Autodesk Inventor part; units mm, degrees
ref_plane "YZ Plane" through (0, 0, 0) normal (1, 0, 0) x (0, 1, 0)
ref_plane "XZ Plane" through (0, 0, 0) normal (0, 1, 0) x (-1, 0, 0)
ref_plane "XY Plane" through (0, 0, 0) normal (0, 0, 1) x (1, 0, 0)
sketch "Sketch1" plane through (0, 0, 0) normal (0, 1, 0) x (-1, 0, 0)
  line L0 (200.4562, 91.842) -> (79.4562, 91.842)
  line L1 (79.4562, 91.842) -> (79.4562, 63.142)
  line L2 (79.4562, 63.142) -> (200.4562, 63.142)
  line L3 (200.4562, 63.142) -> (200.4562, 91.842)
  point P0 (0, 0)
  dimension "d0" = 121
  dimension "d1" = 28.7
extrude "Extrusion1" add sketch "Sketch1" along normal blind 26.8
sketch "Sketch2" plane through (-79.4562, 0, 91.842) normal (1, 0, 0) x (0, 0, -1)
  line L0 (4.95, 3) -> (23.75, 3)
  line L1 (24.75, 4) -> (24.75, 22.8)
  line L2 (23.75, 23.8) -> (4.95, 23.8)
  line L3 (3.95, 22.8) -> (3.95, 4)
  line L4 (28.7, 0) -> (28.7, 26.8)
  line L5 (0, 0) -> (0, 26.8)
  line L6 (0, 26.8) -> (28.7, 26.8)
  arc A0 (24.75, 22.8) -> (23.75, 23.8) centre (23.75, 22.8) ccw
  arc A1 (23.75, 3) -> (24.75, 4) centre (23.75, 4) ccw
  arc A2 (3.95, 4) -> (4.95, 3) centre (4.95, 4) ccw
  arc A3 (4.95, 23.8) -> (3.95, 22.8) centre (4.95, 22.8) ccw
  line L7 (0, 0) -> (28.7, 0)
  point P0 (91.842, 0)
  point P1 (3.95, 3)
  point P2 (24.75, 23.8)
  point P3 (3.95, 23.8)
  dimension "d4" = 20.8
  dimension "d5" = 20.8
  dimension "d7" = 3.95
  dimension "d8" = 3
  dimension "d9" = 1
  dimension "d137" = 3.95
  dimension "d138" = 3
extrude "Extrusion2" cut sketch "Sketch2" against normal blind 121 contours A2 L3 A3 L2 A0 L1 A1 L0
sketch "Sketch3" plane through (0, 0, 0) normal (0, -1, 0) x (1, 0, 0)
  line L0 (-200.4562, 63.142) -> (-200.4562, 91.842)
  line L1 (-200.4562, 91.842) -> (-79.4562, 91.842)
  line L2 (-79.4562, 63.142) -> (-200.4562, 63.142)
  circle A0 centre (-188.2062, 77.492) radius 9.25
  line L3 (-79.4562, 91.842) -> (-79.4562, 63.142)
  point P0 (0, 0)
  dimension "d20" = 14.35
  dimension "d21" = 18.5
  dimension "d287" = 12.25
hole "Hole1" at (-188.2062, 0, 77.492) direction (0, 1, 0) diameter 18.5 depth 5
sketch "Sketch4" plane through (0, 26.8, 0) normal (0, 1, 0) x (1, 0, 0)
  line L0 (-85.9562, -84.142) -> (-193.9562, -84.142)
  line L1 (-193.9562, -84.142) -> (-193.9562, -70.642)
  line L2 (-193.9562, -70.642) -> (-85.9562, -70.642)
  line L3 (-85.9562, -70.642) -> (-85.9562, -84.142)
  line L4 (-79.4562, -91.842) -> (-79.4562, -63.142)
  line L5 (-200.4562, -63.142) -> (-200.4562, -91.842)
  point P0 (0, 0)
  point P1 (-79.4562, -86.142)
  point P2 (-79.4562, -65.142)
  point P3 (-179.4562, -65.142)
  point P4 (-179.4562, -86.142)
  point P5 (-200.4562, -91.842)
  point P6 (-79.4562, -87.892)
  dimension "d30" = 6.5
  dimension "d31" = 6.5
  dimension "d32" = 13.5
  dimension "d41" = 3.75
extrude "Extrusion3" cut sketch "Sketch4" against normal blind 5
sketch "Sketch5" plane through (0, 26.8, 0) normal (0, 1, 0) x (1, 0, 0)
  line L0 (-79.4562, -91.842) -> (-79.4562, -63.142)
  line L1 (-200.4562, -63.142) -> (-200.4562, -91.842)
  line L2 (-79.4562, -91.842) -> (-200.4562, -91.842)
  line L3 (-200.4562, -91.842) -> (-200.4562, -88.442)
  line L4 (-200.4562, -88.442) -> (-79.4562, -88.442)
  line L5 (-79.4562, -88.442) -> (-79.4562, -91.842)
  line L6 (-79.4562, -63.142) -> (-200.4562, -63.142)
  line L7 (-200.4562, -63.142) -> (-200.4562, -66.142)
  line L8 (-200.4562, -66.142) -> (-79.4562, -66.142)
  line L9 (-79.4562, -66.142) -> (-79.4562, -63.142)
  line L10 (-79.4562, -63.142) -> (-200.4562, -63.142)
  line L11 (-79.4562, -87.892) -> (-79.4562, -87.642)
  line L12 (-79.4562, -87.642) -> (-79.4562, -81.492)
  point P0 (0, 0)
  point P1 (-79.4562, -66.142)
  dimension "d38" = 3.4
  dimension "d39" = 3
  dimension "d40" = 0
  dimension "d42" = 22.3
  dimension "d288" = 0.25
  dimension "d289" = 6.15
extrude "Extrusion4" add sketch "Sketch5" along normal blind 8 contours L2 L1 L4 L0 | L1 L6 L0 L8
sketch "Sketch6" plane through (0, 34.8, 0) normal (0, 1, 0) x (1, 0, 0)
  line L0 (-200.4562, -91.842) -> (-79.4562, -91.842)
  line L1 (-200.4562, -66.142) -> (-200.4562, -88.442)
  line L2 (-79.4562, -91.842) -> (-200.4562, -91.842)
  line L3 (-200.4562, -91.842) -> (-200.4562, -84.142)
  line L4 (-200.4562, -84.142) -> (-79.4562, -84.142)
  line L5 (-79.4562, -84.142) -> (-79.4562, -91.842)
  line L6 (-79.4562, -63.142) -> (-200.4562, -63.142)
  line L7 (-79.4562, -63.142) -> (-200.4562, -63.142)
  line L8 (-200.4562, -63.142) -> (-200.4562, -70.642)
  line L9 (-200.4562, -70.642) -> (-79.4562, -70.642)
  line L10 (-79.4562, -70.642) -> (-79.4562, -63.142)
  line L11 (-85.9562, -84.142) -> (-193.9562, -84.142)
  line L12 (-193.9562, -70.642) -> (-85.9562, -70.642)
  point P0 (0, 0)
  point P1 (-200.4562, -91.842)
  dimension "d45" = 0
  dimension "d46" = 0
extrude "Extrusion5" add sketch "Sketch6" along normal blind 3
sketch "Sketch11" plane through (-79.4562, 0, 63.142) normal (0, 0, -1) x (-1, 0, 0)
  line L0 (172.6, 9.3) -> (0, 9.3)
  line L1 (0, 9.3) -> (0, 28.3)
  line L2 (0, 28.3) -> (172.6, 28.3)
  line L3 (172.6, 28.3) -> (172.6, 9.3)
  line L4 (0, 37.8) -> (121, 37.8)
  line L5 (0, 0) -> (0, 37.8)
  line L6 (0, 0) -> (121, 0)
  line L7 (0, 28.3) -> (0, 49.8)
  line L8 (0, 34.8) -> (121, 34.8)
  line L9 (121, 0) -> (121, 37.8)
  point P0 (-79.4562, 0)
  point P1 (0, 3)
  dimension "d97" = 0
  dimension "d105" = 12
  dimension "d110" = 9.5
  dimension "d111" = 21.5
  dimension "d113" = 19
  dimension "d114" = 9.3
  dimension "d174" = 51.6
extrude "Extrusion9" add sketch "Sketch11" along normal blind 26.5 contours L0 L9 L2 L3 | L0 L1 L2 L9
sketch "Sketch12" plane through (-252.0562, 28.3, 63.142) normal (0, 1, 0) x (1, 0, 0)
  line L0 (51.6, 3.25) -> (10.1, 3.25)
  line L1 (10.1, 3.25) -> (10.1, 23.25)
  line L2 (10.1, 23.25) -> (51.6, 23.25)
  line L3 (51.6, 23.25) -> (51.6, 3.25)
  line L4 (0, 0) -> (51.6, 0)
  line L5 (0, 26.5) -> (172.6, 26.5)
  line L6 (0, 0) -> (0, 26.5)
  line L7 (51.6, 0) -> (51.6, -7.5)
  line L8 (172.6, 0) -> (51.6, 0)
  line L9 (172.6, 0) -> (172.6, 26.5)
  point P0 (252.0562, 63.142)
  point P1 (49.2771, 26.5)
  point P2 (51.6, -3.75)
  point P3 (82, 26.5)
  dimension "d120" = 41.5
  dimension "d121" = 20
  dimension "d122" = 3.25
  dimension "d123" = 3.25
  dimension "d127" = 0
  dimension "d128" = 10.1
extrude "Extrusion10" cut sketch "Sketch12" against normal blind 26.5 contours L0 L1 L2 L3
sketch "Sketch14" plane through (-252.0562, 28.3, 63.142) normal (0, 1, 0) x (1, 0, 0)
  circle A0 centre (4.85, 8.25) radius 2.25
  circle A1 centre (4.85, 18.25) radius 2.25
  circle A2 centre (56.85, 8.25) radius 2.25
  circle A3 centre (56.85, 18.25) radius 2.25
  line L0 (10.1, 3.25) -> (10.1, 23.25)
  line L1 (51.6, 23.25) -> (51.6, 3.25)
  line L2 (0, 0) -> (0, 26.5)
  line L3 (51.6, 3.25) -> (10.1, 3.25)
  point P0 (252.0562, 63.142)
  dimension "d141" = 4.5
  dimension "d142" = 4.5
  dimension "d143" = 4.5
  dimension "d144" = 4.5
  dimension "d145" = 5.25
  dimension "d146" = 5.25
  dimension "d148" = 4.85
  dimension "d149" = 5.25
  dimension "d150" = 10
  dimension "d151" = 5
  dimension "d153" = 5.25
  dimension "d154" = 10
  dimension "d155" = 5
sketch "Sketch15" plane through (-252.0562, 9.3, 63.142) normal (-1, 0, 0) x (0, 0, 1)
  line L0 (-23.25, 0) -> (-3.25, 0)
  line L1 (-3.25, 0) -> (-3.25, 14)
  line L2 (-3.25, 14) -> (-23.25, 14)
  line L3 (-23.25, 14) -> (-23.25, 0)
  line L4 (-26.5, 0) -> (-26.5, 19)
  line L5 (0, 0) -> (0, 19)
  line L6 (0, 0) -> (-26.5, 0)
  line L7 (0, 19) -> (-26.5, 19)
  point P0 (-63.142, -9.3)
  dimension "d156" = 3.25
  dimension "d157" = 3.25
  dimension "d158" = 0
  dimension "d159" = 5
extrude "Extrusion11" cut sketch "Sketch15" against normal blind 62 contours L3 L2 L1 L0
hole "Hole3" at (-195.2062, 28.3, 44.892) at (-195.2062, 28.3, 54.892) at (-247.2062, 28.3, 54.892) at (-247.2062, 28.3, 44.892) direction (0, -1, 0) diameter 4.5 depth 6
sketch "Sketch19" plane through (-200.4562, 23.3, 39.892) normal (0, -1, 0) x (1, 0, 0)
  circle A0 centre (5.25, 5) radius 2.25
  line L0 (3.1571, 1.375) -> (1.0642, 5)
  line L1 (1.0642, 5) -> (3.1571, 8.625)
  line L2 (3.1571, 8.625) -> (7.3429, 8.625)
  line L3 (7.3429, 8.625) -> (9.4358, 5)
  line L4 (9.4358, 5) -> (7.3429, 1.375)
  line L5 (7.3429, 1.375) -> (3.1571, 1.375)
  circle A1 centre (5.25, 15) radius 2.25
  line L6 (3.1571, 11.375) -> (1.0642, 15)
  line L7 (1.0642, 15) -> (3.1571, 18.625)
  line L8 (3.1571, 18.625) -> (7.3429, 18.625)
  line L9 (7.3429, 18.625) -> (9.4358, 15)
  line L10 (9.4358, 15) -> (7.3429, 11.375)
  line L11 (7.3429, 11.375) -> (3.1571, 11.375)
  circle A2 centre (-46.75, 5) radius 2.25
  line L12 (-50.9358, 5) -> (-48.8429, 8.625)
  line L13 (-48.8429, 8.625) -> (-44.6571, 8.625)
  line L14 (-44.6571, 8.625) -> (-42.5642, 5)
  line L15 (-42.5642, 5) -> (-44.6571, 1.375)
  line L16 (-44.6571, 1.375) -> (-48.8429, 1.375)
  line L17 (-48.8429, 1.375) -> (-50.9358, 5)
  circle A3 centre (-46.75, 15) radius 2.25
  line L18 (-50.9358, 15) -> (-48.8429, 18.625)
  line L19 (-48.8429, 18.625) -> (-44.6571, 18.625)
  line L20 (-44.6571, 18.625) -> (-42.5642, 15)
  line L21 (-42.5642, 15) -> (-44.6571, 11.375)
  line L22 (-44.6571, 11.375) -> (-48.8429, 11.375)
  line L23 (-48.8429, 11.375) -> (-50.9358, 15)
  line L24 (0, 0) -> (0, 20)
  line L25 (0, 0) -> (0, 20)
  line L26 (10.4, 0) -> (0, 0)
  line L27 (0, 0) -> (0, 20)
  line L28 (0, 20) -> (10.4, 20)
  line L29 (10.4, 20) -> (10.4, 0)
  line L30 (-51.6, 0) -> (-51.6, 20)
  line L31 (-41.5, 0) -> (-51.6, 0)
  line L32 (-51.6, 0) -> (-51.6, 20)
  line L33 (-51.6, 20) -> (-41.5, 20)
  line L34 (-41.5, 20) -> (-41.5, 0)
  point P0 (200.4562, -39.892)
  point P1 (5.25, 15)
  point P2 (-51.6, 0)
  dimension "d191" = 7.25
  dimension "d194" = 7.25
  dimension "d197" = 0
  dimension "d198" = 0
  dimension "d199" = 7.25
  dimension "d200" = 7.25
extrude "Extrusion14" add sketch "Sketch19" along normal blind 6 contours L24 L28 L29 L26 | L30 L33 L34 L31
fillet "Fillet8" radius 2 2 edges at (-200.4562, 28.3, 49.892) (-241.9562, 28.3, 49.892)
sketch "Sketch25" plane through (-200.4562, 0, 91.842) normal (0, 0, 1) x (1, 0, 0)
  line L0 (0, 27.8) -> (12.25, 27.8)
  line L1 (12.25, 27.8) -> (12.25, 10)
  line L2 (12.25, 10) -> (0, 10)
  line L3 (0, 10) -> (0, 27.8)
  line L4 (0, 0) -> (0, 37.8)
  line L5 (0, 37.8) -> (121, 37.8)
  line L6 (0, 0) -> (121, 0)
  line L7 (108.75, 27.8) -> (121, 27.8)
  line L8 (121, 27.8) -> (121, 10)
  line L9 (121, 10) -> (108.75, 10)
  line L10 (108.75, 10) -> (108.75, 27.8)
  line L11 (121, 0) -> (121, 37.8)
  point P0 (200.4562, 0)
  dimension "d250" = 0
  dimension "d251" = 37.8
  dimension "d252" = 10
  dimension "d253" = 10
  dimension "d254" = 0
  dimension "d255" = 10
  dimension "d256" = 10
  dimension "d257" = 12.25
  dimension "d258" = 12.25
extrude "Extrusion18" add sketch "Sketch25" along normal blind 12.25 contours L0 L1 L2 L3
extrude "Extrusion19" add sketch "Sketch25" along normal blind 12.25 contours L8 L9 L10 L7
sketch "Sketch26" plane through (-200.4562, 27.8, 91.842) normal (0, 1, 0) x (1, 0, 0)
  circle A0 centre (6.125, -6.125) radius 3.125
  line L0 (12.25, 0) -> (12.25, -12.25)
  line L1 (12.25, -12.25) -> (0, -12.25)
  circle A1 centre (114.875, -6.125) radius 3.125
  line L2 (121, 0) -> (121, -12.25)
  line L3 (121, -12.25) -> (108.75, -12.25)
  point P0 (200.4562, 91.842)
  dimension "d263" = 6.25
  dimension "d266" = 6.125
  dimension "d267" = 6.125
  dimension "d268" = 6.25
  dimension "d269" = 6.125
  dimension "d270" = 6.125
hole "Hole5" at (-194.3312, 27.8, 97.967) at (-85.5812, 27.8, 97.967) direction (0, -1, 0) diameter 6.25 depth 20
sketch "Sketch28" plane through (-252.0562, 28.3, 63.142) normal (0, 1, 0) x (1, 0, 0)
  line L0 (172.6, 0) -> (172.6, 26.5)
  line L1 (62, 3.25) -> (62, 23.25)
  line L2 (0, 3.25) -> (62, 3.25)
  line L3 (172.6, 0) -> (172.6, 26.5)
  line L4 (172.6, 26.5) -> (172.6, 0)
  line L5 (172.6, 26.5) -> (62, 26.5)
  line L6 (0, 26.5) -> (172.6, 26.5)
  line L7 (62, 26.5) -> (172.6, 0)
  line L8 (62, 23.25) -> (158.9481, 0)
  line L9 (172.6, 0) -> (51.6, 0)
  line L10 (62, 3.25) -> (145.3962, 3.25)
  point P0 (252.0562, 63.142)
extrude "Extrusion20" cut sketch "Sketch28" against normal blind 30
fillet "Fillet12" radius 1 1 edges at (-190.0562, 18.8, 36.642)
fillet "Fillet13" radius 0.5 1 edges at (-139.9562, 34.8, 88.442)
fillet "Fillet14" radius 0.5 1 edges at (-139.9562, 26.8, 88.442)
properties part number "shaftHolder4V1"
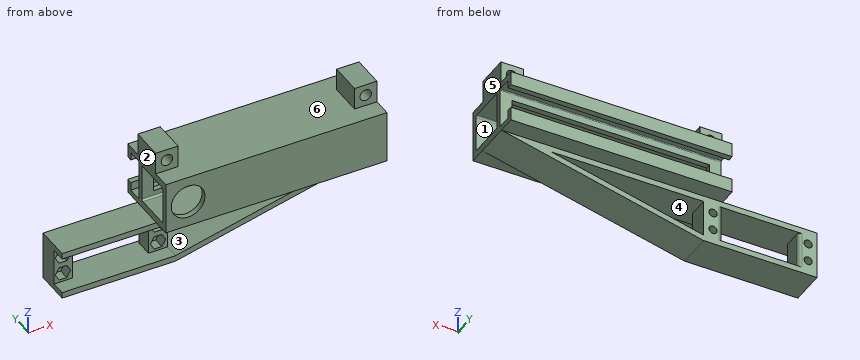
The model under review builds one solid part; all positions refer to its coordinate system, in mm. Face numbers are marked on the shaded views. A direction names the side the tool comes from. Round coordinates to 2 decimals unless told otherwise and drop trailing zeros. Loops run counter-clockwise (first coordinate to the right, second up) from the corner with the lowest first, then second, coordinate; pieces in that order, holes last. Notation, with made-up numbers: (-28, -9) -> (26, -9) arc R21 ccw to (26, 28) -> close; hole circle Ø1 at (52.5, 65). An arc over 180 degrees is marked (long way). Answer as CSV lines item,"result".
1) For P1, Ø6, axis at x = -122.5, y = 25.5, coming from the -Z side; P2, Ø9.5, axis at x = -149.5, z = 77.5, coming from the +Y side; P3, Ø2.5, axis at x = -140.5, y = 30, coming from the +Z side, all flat-tipped, find the tip position at first contact; note any pin that passes through.
Geometry results:
P1,"stops at z = 52.11"
P2,"stops at y = 3"
P3,"stops at z = 91.84"
2) Add section D-D on y = 13. Write out the cut boundary in (x, z) (3 decimals), plus the area to 3 significant figures.
Geometry results:
outline,"(-252.056, 36.642) -> (-190.174, 36.642) arc R1 ccw to (-189.941, 36.67) -> (-79.456, 63.142) -> (-79.456, 67.092) -> (-200.456, 67.092) -> (-200.456, 63.142) -> (-252.056, 63.142) -> (-252.056, 59.892) -> (-106.66, 59.892) -> (-190.056, 39.892) -> (-252.056, 39.892) -> close; (-200.456, 87.892) -> (-79.456, 87.892) -> (-79.456, 104.092) -> (-91.706, 104.092) -> (-91.706, 91.842) -> (-188.206, 91.842) -> (-188.206, 104.092) -> (-200.456, 104.092) -> close; hole circle Ø6.25 at (-194.331, 97.967); hole circle Ø6.25 at (-85.581, 97.967)"
area,"2,230 mm²"
3) Add section B-B on x = -225.5. Write out the cut boundary in (y, z), plus the area to 4 significant figures.
Geometry results:
outline,"(9.3, 36.64) -> (28.3, 36.64) -> (28.3, 39.89) -> (9.3, 39.89) -> close; (9.3, 59.89) -> (28.3, 59.89) -> (28.3, 63.14) -> (9.3, 63.14) -> close"
area,"123.5 mm²"
4) Tool access review of the marked faces 1, 2 and 3: name each direction out of +Z, -Z, +X, -X, +Y, -Y from which nothing blocks a thin tool from reaching the whole face with its end or side.
Geometry results:
face 1,"+X, -X"
face 2,"+Z, -X, +Y, -Y"
face 3,"+Y, -Y"
5) Add section A-A on y = 32. Write out the cut boundary in (x, z).
Geometry results:
outline,"(-200.46, 63.14) -> (-79.46, 63.14) -> (-79.46, 66.14) -> (-200.46, 66.14) -> close; (-200.46, 88.44) -> (-79.46, 88.44) -> (-79.46, 91.84) -> (-200.46, 91.84) -> close"
6) To check wall thickness, follow line 1 along Z through (x, y) = (-139.5, 36.5); line 2 along Z through (x, y) = (-199, 14); line 3 along Z through (x, y) = (-170.5, 32). State the ranges of each line that lie inside material, in increasing order. Write a range as from..to.
Geometry results:
line 1,"z = 63.14..70.64, 84.14..91.84"
line 2,"z = 36.64..39.89, 59.89..67.09, 87.89..104.09"
line 3,"z = 63.14..66.14, 88.44..91.84"
7) Draft analysis for pull direction Z (two halves, no side actions). For the marked faces 4, 5 and 6, state which applies: pulls with the +Z half, pulls with the -Z half, needs draft (parallel to the pull), parting line crosses it, or undercut.
Geometry results:
face 4,"undercut"
face 5,"needs draft"
face 6,"pulls with the +Z half"
8) Add section C-C on z = 99. Write out the cut boundary in (x, y).
Geometry results:
outline,"(-200.46, 10) -> (-197.28, 10) -> (-197.28, 27.8) -> (-200.46, 27.8) -> close; (-191.38, 10) -> (-188.21, 10) -> (-188.21, 27.8) -> (-191.38, 27.8) -> close; (-91.71, 10) -> (-88.53, 10) -> (-88.53, 27.8) -> (-91.71, 27.8) -> close; (-82.63, 10) -> (-79.46, 10) -> (-79.46, 27.8) -> (-82.63, 27.8) -> close"
